Could you check a few things on this model? Use its own coordinates, in mm. Face numbers are marked on the shaded views. A direction names the side the tool comes from. Give positions to 0.01 mm unless a question says otherwise; leave off trailing zeros. Loops run counter-clockwise (first coordinate to the right, second up) from the corner with the lowest first, then second, coordinate; pieces in that order, holes last. Notation, with made-up numbers: (70, 17.5) - (101, 17.5) arc R27 ccw to (101, 40.5) - close; hole circle Ø5 at (7, 41). An arc over 180 degrees is marked (long way). Write each question's results on one line, items separated by ' | '. Start each with the question number.
1) I want a section at A-A, the plane x = 3.25. Write out the boundary of the cut face in (y, z).
2) I want a section at C-C, the plane y = -1. Count the separate pieces of the cut face and the enclosed holes in it, and give its area (3 significant figures).
3) I want a section at B-B, the plane x = -10. Write out the boundary of the cut face in (y, z).
4) If I drill on probe 1 along Y at (x, z) = (0.25, 1.5); probe 2 along X at (y, z) = (2.25, 2.5); probe 3 along Y at (x, z) = (-9, 4.5), over which ranges is the centre line in solid material (lowest first)? Write a range as [from, to].
5) On a 3-axis mill with a long thin cutter (end or side, diameter ignored), from which of +Z, -Z, +X, -X, +Y, -Y can I reach the whole of each face in a straight line? I mean the marked faces 4, 5, 6 and 7. Say none if no direction works.
6) If we mould it in two halves opening along X, with no side actions, what happens to the marked faces 1, 2 and 3? For each: +X half, -X half, draft (parallel to the pull), parting line (faces both ways), or undercut.
7) I'm going to push flat-ended pins straight in: pin 1 (2 mm diameter, centred on x = -8.5, z = 4.5, fed in from +Y); pin 2 (3.5 mm diameter, centred on x = -10, z = 5, fed in from -Y); pin 3 (3.5 mm diameter, centred on y = 0, z = 4.5, fed in from -X). Where does each tip first touch, or does it pass through?
from build123d import *

# Parameters (mm, degrees)
F0_W     = 13.1
F0_H     = 13.1
F0_W_2   = 9.5
F0_H_2   = 9.5
F1_DEPTH = 9
F3_DEPTH = 5
F5_R     = 3
F5_R_2   = 1.5
F6_DEPTH = 2
F8_DEPTH = 25
F9_R     = 0.9


with BuildPart() as f1:
    # F0 (on Top) → F1 (new body)
    with BuildSketch(Plane.XY):
        Rectangle(F0_W, F0_H)
        Rectangle(F0_W_2, F0_H_2, mode=Mode.SUBTRACT)
    extrude(amount=F1_DEPTH)

    # F2 (on Front) → F3 (join, symmetric)
    with BuildSketch(Plane.XZ):
        Polygon((-6.55, 0), (-6.55, 4.5), (-9.55, 4.5), (-9.55, 6.775), (-11.05, 6.775), (-11.05, 4.5), (-12.85, 4.5), (-12.85, 6.775), (-14.35, 6.775), (-14.35, 2.975), align=None)
        Polygon((-9.55, 4.5), (-6.55, 4.5), (-6.55, 9), (-14.35, 9), (-14.35, 6.775), (-12.85, 6.775), (-12.85, 4.5), (-11.05, 4.5), (-11.05, 6.775), (-9.55, 6.775), align=None)
        Polygon((-14.35, 0), (-6.55, 0), (-14.35, 2.975), align=None)
    extrude(amount=F3_DEPTH, both=True)

    # F5 (on offset) → F6 (cut)
    with BuildSketch(Plane.XY.offset(9)):
        with Locations((-10, 0)):
            Circle(F5_R)
        with Locations((-10, 0)):
            Circle(F5_R_2, mode=Mode.SUBTRACT)
    extrude(amount=-F6_DEPTH, mode=Mode.SUBTRACT)

    # F7 (on Right) → F8 (cut)
    with BuildSketch(Plane.YZ):
        with BuildLine():
            ThreePointArc((0, 2.5), (1.4142135624, 3.0857864376), (2, 4.5))
            ThreePointArc((2, 4.5), (-1.4142135624, 5.9142135624), (0, 2.5))
        make_face()
    extrude(amount=-F8_DEPTH, mode=Mode.SUBTRACT)

    # F9
    f9_edges = [f1.edges().sort_by_distance(p)[0] for p in [
        (-14.35, 0, 9),
        (-14.35, 5, 4.5),
        (-14.35, -5, 4.5),
        (-14.35, 0, 0),
        (-14.35, 0, 6.5),
        (-6.55, 6.55, 4.5),
        (6.55, 6.55, 4.5),
        (-6.55, -6.55, 4.5),
        (-10.45, 5, 9),
        (-10.45, 5, 0),
        (6.55, -6.55, 4.5),
        (-10.45, -5, 0),
        (-10.45, -5, 9),
    ]]
    fillet(f9_edges, radius=F9_R)


solid = f1.part
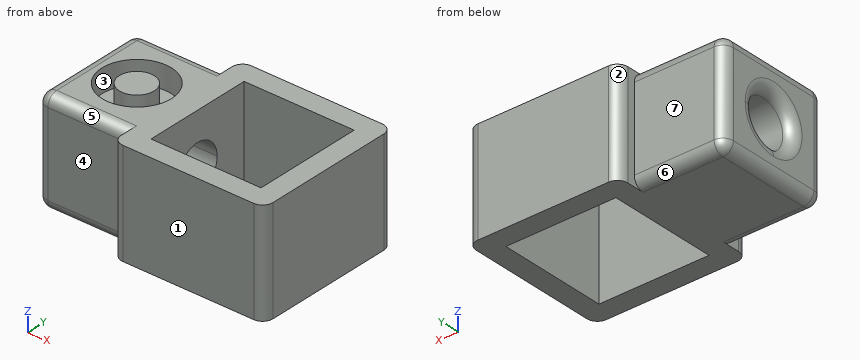
Answers:
1) outline: (-6.55, 0) - (-4.75, 0) - (-4.75, 9) - (-6.55, 9) - close; (4.75, 0) - (6.55, 0) - (6.55, 9) - (4.75, 9) - close
2) separate pieces: 3 | enclosed holes: 0 | area: 61.8 mm2
3) outline: (-5, 0.9) arc R0.9 ccw to (-4.1, 0) - (4.1, 0) arc R0.9 ccw to (5, 0.9) - (5, 8.1) arc R0.9 ccw to (4.1, 9) - (3, 9) - (3, 7) - (1.5, 7) - (1.5, 9) - (-1.5, 9) - (-1.5, 7) - (-3, 7) - (-3, 9) - (-4.1, 9) arc R0.9 ccw to (-5, 8.1) - close; hole circle Ø4 at (0, 4.5)
4) probe 1: y = [-6.55, -4.75], [4.75, 6.55] | probe 2: x = [-14.35, -4.75], [4.75, 6.55] | probe 3: y = [-5, -2], [2, 5]
5) face 4: +Z, -Z, -X, -Y | face 5: +Z, -X, -Y | face 6: -Z, -X, +Y | face 7: +Z, -Z, -X, +Y
6) face 1: draft | face 2: -X half | face 3: undercut
7) pin 1: stops at y = 5 | pin 2: stops at y = -5 | pin 3: stops at x = 4.75
